Could you check a few things on this model? Use its own coordinates, in mm. A direction names the side the tool comes from. Give positions to 0.01 mm unless a question says otherwise; leave off trailing zeros. Loops run counter-clockwise (first coordinate to the right, second up) from the corner with the lowest first, then second, coordinate; pieces in that order, holes last. Notation, with made-up numbers: M -40,-20.5 L 11,-20.5 A32 cw 11,17.5 Z; hole C 43.25,-25 d8. An arc over 180 degrees is marked long. Answer in a Markdown table with one row per item. Add a question column.
1. If we section it at B-B on y = 13: List the corners of the cut face in (x, z) for me, then the cut area to 3 significant figures.
2. If we section it at A-A on z = 1.15: List the corners of the cut face in (x, y) for me.
3. I need wall thicknesses on line 1 along Y through (x, z) = (-0.75, 1.65); line 2 along X through (y, z) = (20.5, 0.2); line 3 along X through (y, z) = (14, 1.6). Which ranges of each line are inside material? Lowest first, please. Write a range as from..to.
4. If we section it at D-D on y = 11.25: List the corners of the cut face in (x, z) for me.
5. Thinking about a two-plate mould opening in X: for faces 1 (the flat face through (-2.5, 21, 1)), 2 (the cylindrical face through (-0.325, 11.536, 1.014)), 3 (the flat face through (3.9, 17, 1)), which applies, released by +X, released by -X, zero draft, split by the parting line, or undercut?
6. If we section it at C-C on x = 2: List the corners of the cut face in (y, z) for me, then the cut area to 3 significant figures.
7. Which directions (+Z, -Z, +X, -X, +Y, -Y) give clear straight access to the entire face, cutting with the end or side of a thin tool? Please do faces 4 (the flat face through (2.5, 21, 1)), 5 (the cylindrical face through (-3.21, 19.74, 0.99)).
8. I'm going to push a flat-ended pin straight in: pin 1 Ø0.6 at (y, z) = (20.5, 0.5) entering from -X. Where does the tip first touch, or does it pass through?
Autodesk Inventor part; units mm, degrees
ref_plane "YZ Plane" through (0, 0, 0) normal (1, 0, 0) x (0, 1, 0)
ref_plane "XZ Plane" through (0, 0, 0) normal (0, 1, 0) x (-1, 0, 0)
ref_plane "XY Plane" through (0, 0, 0) normal (0, 0, 1) x (1, 0, 0)
sketch "스케치1" plane through (0, 0, 0) normal (0, 0, 1) x (1, 0, 0)
  circle A0 centre (0, 0) radius 20
  line L0 (-3.9, 19.6161) -> (-3.9, 0)
  line L1 (-3.9, 0) -> (3.9, 0)
  line L2 (3.9, 0) -> (3.9, 19.6161)
  circle A1 centre (0, 0) radius 10
  line L3 (-2.5, 21.8575) -> (-2.5, 19.8431)
  line L4 (2.5, 21.8575) -> (2.5, 19.8431)
  circle A2 centre (0, 0) radius 22
  point P0 (0, 0)
  point P1 (0, 0)
  point P2 (-3.9, 9.2081)
  point P3 (3.9, 9.2081)
  dimension "d0" = 40
  dimension "d1" = 7.8
  dimension "d5" = 20
  dimension "d13" = 2
  dimension "d14" = 5
  dimension "d15" = 2.5
extrude "돌출1" add sketch "스케치1" along normal blind 2 contours L2 A1 L0 A0 | A0 L3 A2 L4 picked at (1.4966, 13.2144) picked at (-1.9451, 20.5611)
sketch "스케치2" plane through (0, 0, 2) normal (0, 0, 1) x (1, 0, 0)
  circle A0 centre (0, 13) radius 1.5
  arc A1 (3.9, 9.2081) -> (-3.9, 9.2081) centre (0, 0) ccw
  point P0 (0, 0)
  point P1 (0, 10)
  dimension "d6" = 3
  dimension "d7" = 3
extrude "돌출2" cut sketch "스케치2" against normal through all
fillet "모깎기1" radius 3.8 2 edges at (-3.9, 9.2081, 1) (3.9, 9.2081, 1)
properties part number "ModuleConnector_Outside_Axis_3D 인쇄"
Results:
| question | item | result |
|---|---|---|
| 1 | outline | M -3.81,0 L -1.5,0 L -1.5,2 L -3.81,2 Z; M 1.5,0 L 3.81,0 L 3.81,2 L 1.5,2 Z |
| 1 | area | 9.26 mm2 |
| 2 | outline | M -3.9,13.8 A3.8 ccw -0.07,10 A10 cw 0.07,10 A3.8 ccw 3.9,13.8 L 3.9,19.62 A20 ccw 2.5,19.84 L 2.5,21.86 A22 ccw -2.5,21.86 L -2.5,19.84 A20 ccw -3.9,19.62 Z; hole C 0,13 d3 |
| 3 | line 1 | 10.06..11.7, 14.3..21.99 |
| 3 | line 2 | -2.5..2.5 |
| 3 | line 3 | -3.9..-1.12, 1.12..3.9 |
| 4 | outline | M -2.92,0 L 2.92,0 L 2.92,2 L -2.92,2 Z |
| 5 | face 1 | released by -X |
| 5 | face 2 | undercut |
| 5 | face 3 | released by +X |
| 6 | outline | M 10.51,0 L 21.91,0 L 21.91,2 L 10.51,2 Z |
| 6 | area | 22.8 mm2 |
| 7 | face 4 | +Z, -Z, +X, +Y |
| 7 | face 5 | +Z, -Z, -X, +Y |
| 8 | pin 1 | x = -2.5 |
